Work out the finished part from the listing and answer in its coordinate system (mm). A direction names the side the tool comes from. Coordinates: 2 decimals unless noted, no trailing zeros. Order: outer loops, then holes, each group sorted by start corner. A loop starts at its lowest first (then second) coordinate and runs counter-clockwise, first axis right, second up.
```python
from build123d import *

# Parameters (mm, degrees)
SKETCH1_W                      = 2.1
SKETCH1_H                      = 8
REVOLVE1_ANGLE                 = 180
SKETCH2_W                      = 2.1
SKETCH2_H                      = 16
BOSS_EXTRUDE1_DEPTH            = 13.2
BOSS_EXTRUDE2_DEPTH            = 2.1
F_4_2_4_2_DIAMETER_HOLE1_D     = 4.2
F_4_2_4_2_DIAMETER_HOLE1_DEPTH = 23.3


with BuildPart() as part:
    # Sketch1 → Revolve1 (revolve)
    with BuildSketch(Plane(origin=(0, 0, 15.3), x_dir=(-1, 0, 0), z_dir=(0, 0, -1))):
        with Locations((-1.05, 12)):
            Rectangle(SKETCH1_W, SKETCH1_H)
    revolve(axis=Axis((2.1, 8, 15.3), (1, 0, 0)), revolution_arc=REVOLVE1_ANGLE)

    # Sketch2 → Boss-Extrude1 (add)
    with BuildSketch(Plane(origin=(0, 0, 15.3), x_dir=(-1, 0, 0), z_dir=(0, 0, -1))):
        with Locations((-1.05, 8)):
            Rectangle(SKETCH2_W, SKETCH2_H)
    extrude(amount=BOSS_EXTRUDE1_DEPTH)

    # Sketch3 → Boss-Extrude2 (add)
    with BuildSketch(Plane(origin=(0, 0, 2.1), x_dir=(-1, 0, 0), z_dir=(0, 0, -1))):
        with BuildLine():
            Line((-15.4, 16), (0, 16))
            Line((0, 16), (0, 0))
            Line((0, 0), (-15.4, 0))
            ThreePointArc((-15.4, 0), (-23.4, 8), (-15.4, 16))
        make_face()
    extrude(amount=BOSS_EXTRUDE2_DEPTH)

    # Ø4.2 (4.2) Diameter Hole1
    with Locations(Plane(origin=(0, 0, 0), x_dir=(-1, 0, 0), z_dir=(0, 0, -1))):
        with Locations((-14.1, 8)):
            Hole(F_4_2_4_2_DIAMETER_HOLE1_D / 2, depth=F_4_2_4_2_DIAMETER_HOLE1_DEPTH)


solid = part.part
```
1. Flat-ended cylindrical pins translate along their axes: pin 1 (8 mm diameter, centred on x = 13.5, z = 6.5, fed in from +Y); pin 2 (1 mm diameter, centred on y = 13.5, z = 11.5, fed in from +X); pin 3 (6.5 mm diameter, centred on x = 14.1, y = 8, fed in from +Z). Find the tip coordinate at first contact, or state that the pin passes through.
2. The part is cut by section B-B (y = 8). Determine the outline of the cut face in (x, z), plus the area to 3 significant figures.
3. The part is cut by section A-A (x = 14.1). Determine the outline of the cut face in (y, z).
4. For faces 4 (the cylindrical face through (1.035, 8.176, 23.298)), 5 (the flat face through (10, 8, 2.1)), determine the directions among +Z, -Z, +X, -X, +Y, -Y from which every point of the face is accessible in a straight line to the end or side of a thin tool.
5. The part is cut by section C-C (z = 11.5). Determine the outline of the cut face in (x, y).
6. The part is cut by section D-D (y = 13.25). Determine the outline of the cut face in (x, z), plus the area to 3 significant figures.
7. The mould has two halves that part along Y. Classify faces 1 (the cylindrical face through (12.552, 9.419, 1.065)), 2 (the cylindrical face through (23.398, 7.824, 1.065)), 3 (the flat face through (0, 8, 12)): released by +Y, released by -Y, zero draft, split by the parting line, or undercut.
8. Consider probe 1 along Y at (x, z) = (14.1, 1.7); probe 2 along Z at (x, y) = (7.75, 9.75). Determine where each line is inside the solid, lowest interval first.
Worked out:
1. pin 1: passes through
1. pin 2: stops at x = 2.1
1. pin 3: stops at z = 2.1
2. outline: (0, 0) - (12, 0) - (12, 2.1) - (2.1, 2.1) - (2.1, 23.3) - (0, 23.3) - close; (16.2, 0) - (23.4, 0) - (23.4, 2.1) - (16.2, 2.1) - close
2. area: 84.8 mm2
3. outline: (0, 0) - (5.9, 0) - (5.9, 2.1) - (0, 2.1) - close; (10.1, 0) - (16, 0) - (16, 2.1) - (10.1, 2.1) - close
4. face 4: +Z, +X, -X
4. face 5: +Z, +X, +Y, -Y
5. outline: (0, 0) - (2.1, 0) - (2.1, 16) - (0, 16) - close
6. outline: (0, 0) - (21.44, 0) - (21.44, 2.1) - (2.1, 2.1) - (2.1, 21.34) - (0, 21.34) - close
6. area: 85.4 mm2
7. face 1: undercut
7. face 2: split by the parting line
7. face 3: zero draft
8. probe 1: y = 0 to 5.9, 10.1 to 16
8. probe 2: z = 0 to 2.1
